Source: CAD feature listing. Evaluate the final solid. Frame: model axes, mm. A direction names the side the tool comes from. Give positions to 0.01 mm unless a question says otherwise; leave off trailing zeros. Order: outer loops, then holes, each group sorted by start corner. A loop starts at its lowest first (then second) coordinate and runs counter-clockwise, first axis right, second up. Notation, with made-up numbers: (72, 37) - (109, 37) arc R8 ccw to (109, 44) - close; hole circle Ø5 at (-9.5, -2). An arc over 180 degrees is marked (long way). One line per item, written item: value. Start each with the question number.
from build123d import *

# Parameters (mm, degrees)
BASE_FLANGE1_DEPTH = 25.4
SKETCH3_R          = 2.3876
CUT_EXTRUDE1_DEPTH = 5.08
SKETCH4_R          = 2.3876
CUT_EXTRUDE2_DEPTH = 5.08


# Sheet-metal steps are written as plain solids
with BuildPart() as part:
    # Sketch1 → Base-Flange1 (new body)
    with BuildSketch(Plane.XY):
        with BuildLine():
            Line((76.2, 0), (4.7752, 0))
            ThreePointArc((4.7752, 0), (1.398623698, -1.398623698), (0, -4.7752))
            Line((0, -4.7752), (0, -76.2))
            Line((0, -76.2), (3.175, -76.2))
            Line((3.175, -76.2), (3.175, -4.7752))
            ThreePointArc((3.175, -4.7752), (3.643687729, -3.643687729), (4.7752, -3.175))
            Line((4.7752, -3.175), (76.2, -3.175))
            Line((76.2, -3.175), (76.2, 0))
        make_face()
    extrude(amount=-BASE_FLANGE1_DEPTH)

    # Sketch3 → Cut-Extrude1 (cut)
    with BuildSketch(Plane(origin=(0, 0, 0), x_dir=(-1, 0, 0), z_dir=(0, 1, 0))):
        with Locations(Location((-66.675, -12.7, 0), (0, 0, 90))):
            Circle(SKETCH3_R)
        with Locations(Location((-38.1, -12.7, 0), (0, 0, 90))):
            Circle(SKETCH3_R)
    extrude(amount=-CUT_EXTRUDE1_DEPTH, mode=Mode.SUBTRACT)

    # Sketch4 → Cut-Extrude2 (cut)
    with BuildSketch(Plane.ZY):
        with Locations(Location((-12.7, -66.675, 0), (0, 0, 270))):
            Circle(SKETCH4_R)
        with Locations(Location((-12.7, -38.1, 0), (0, 0, 270))):
            Circle(SKETCH4_R)
    extrude(amount=-CUT_EXTRUDE2_DEPTH, mode=Mode.SUBTRACT)


solid = part.part
1. Section A-A on z = -12.7. Return the cut outline in (x, y) (3 decimals), then the cut area to 3 significant figures.
2. Section C-C on x = 38.1. Return the cut outline in (y, z) (3 decimals).
3. Section B-B on y = -38.1. Return the cut outline in (x, z) (3 decimals), then the cut area to 3 significant figures.
4. Ray query, L1, parallel to X at y = -1.15, z = -12.7; L2, parallel to X at y = -2.2, z = -12.7; L3, parallel to Y at x = 70, z = -1.5 (3 decimals). Return the intervals inside material, ascending.
5. Draft query along X for faces 1 (the cylindrical face through (1.565, -36.205, -14.153)), 2 (the cylindrical face through (1.4, -1.4, -12.5)), 3 (the cylindrical face through (37.186, -1.565, -10.494)). Return one class per face: pulls with the +X half, pulls with the -X half, needs draft (parallel to the pull), parting line crosses it, or undercut.
6. Set-up query: faces 4 (the flat face through (40, -3.175, -15)), 5 (the cylindrical face through (1.57, -68.95, -11.98)). Return all of +Z, -Z, +X, -X, +Y, -Y with unobstructed straight access to the full face (end or side cutting, diameter ignored); none if empty.
7. Contact query for flat-ended pins moving along their axis: pin 1 Ø12.5 at (x, z) = (52, -13.5) entering from -Y (3 decimals); pin 2 Ø2 at (y, z) = (-42.5, -17) entering from +X (3 decimals); pin 3 Ø4 at (y, z) = (-38.1, -12.7) entering from +X. Output: stop coordinate, or through.
8. Section D-D on z = -6. Return the cut outline in (x, y) (3 decimals), then the cut area to 3 significant figures.
Data:
1. outline: (0, -76.2) - (3.175, -76.2) - (3.175, -69.063) - (0, -69.063) - close; (0, -64.287) - (3.175, -64.287) - (3.175, -40.488) - (0, -40.488) - close; (0, -35.712) - (3.175, -35.712) - (3.175, -4.775) arc R1.6 cw to (4.775, -3.175) - (35.712, -3.175) - (35.712, 0) - (4.775, 0) arc R4.775 ccw to (0, -4.775) - close; (40.488, -3.175) - (64.287, -3.175) - (64.287, 0) - (40.488, 0) - close; (69.063, -3.175) - (76.2, -3.175) - (76.2, 0) - (69.063, 0) - close
1. area: 409 mm2
2. outline: (-3.175, -25.4) - (0, -25.4) - (0, -15.088) - (-3.175, -15.088) - close; (-3.175, -10.312) - (0, -10.312) - (0, 0) - (-3.175, 0) - close
3. outline: (0, -25.4) - (3.175, -25.4) - (3.175, -15.088) - (0, -15.088) - close; (0, -10.312) - (3.175, -10.312) - (3.175, 0) - (0, 0) - close
3. area: 65.5 mm2
4. L1: x = 1.67 to 35.71, 40.49 to 64.29, 69.06 to 76.2
4. L2: x = 0.75 to 35.71, 40.49 to 64.29, 69.06 to 76.2
4. L3: y = -3.175 to 0
5. face 1: needs draft
5. face 2: pulls with the -X half
5. face 3: undercut
6. face 4: +Z, -Z, +X, -Y
6. face 5: +X, -X
7. pin 1: stops at y = -3.175
7. pin 2: stops at x = 3.175
7. pin 3: passes through
8. outline: (0, -76.2) - (3.175, -76.2) - (3.175, -4.775) arc R1.6 cw to (4.775, -3.175) - (76.2, -3.175) - (76.2, 0) - (4.775, 0) arc R4.775 ccw to (0, -4.775) - close
8. area: 469 mm2
